Work out the finished part from the listing and answer in its coordinate system (mm). Face numbers are marked on the shaded views. A direction names the side the tool comes from. Coordinates: 2 decimals unless noted, no trailing zeros. Loops run counter-clockwise (first coordinate to the right, second up) from the corner with the lowest first, then second, coordinate; pieces in that order, holes last. Notation, with made-up numbers: (67, 88) -> (73, 88) arc R18 cw to (73, 112) -> close; hole circle Ø2 at (56.25, 11). An arc over 180 degrees is marked (long way). Answer as CSV lines item,"result".
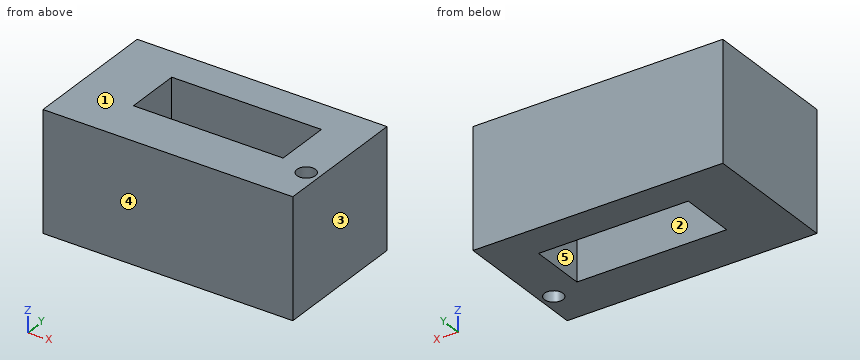
```python
from build123d import *

# Parameters (mm, degrees)
F0_W     = 53.355787
F0_H     = 29.385667
F0_R     = 1.970291
F0_W_2   = 31.967147
F0_H_2   = 11.958933
F1_DEPTH = 25.4


with BuildPart() as f1:
    # F0 (on Top) → F1 (new body)
    with BuildSketch(Plane.XY):
        with Locations((26.677893, 14.692833)):
            Rectangle(F0_W, F0_H)
        with Locations((50.581049, 8.259824)):
            Circle(F0_R, mode=Mode.SUBTRACT)
        with Locations((28.403014, 16.046856)):
            Rectangle(F0_W_2, F0_H_2, mode=Mode.SUBTRACT)
    extrude(amount=F1_DEPTH)


solid = f1.part
```
(1) A cutting plane is placed at B-B, the plane x = 41. Write down the section's boundary in (y, z), and give its area (3 significant figures).
Computed values:
outline,"(0, 0) -> (10.07, 0) -> (10.07, 25.4) -> (0, 25.4) -> close; (22.03, 0) -> (29.39, 0) -> (29.39, 25.4) -> (22.03, 25.4) -> close"
area,"443 mm2"
(2) Consider line 1 along Y through (x, z) = (19, 5.75); line 2 along X through (y, z) = (21.5, 20.5); line 3 along X through (y, z) = (8.75, 15.5). Determine where each line is inside the solid, lowest interval first.
Computed values:
line 1,"0 to 10.07, 22.03 to 29.39"
line 2,"0 to 12.42, 44.39 to 53.36"
line 3,"0 to 48.67, 52.49 to 53.36"
(3) A cutting plane is placed at C-C, the plane z = 15. Write down the section's boundary in (x, y).
Computed values:
outline,"(0, 0) -> (53.36, 0) -> (53.36, 29.39) -> (0, 29.39) -> close; hole (12.42, 10.07) -> (44.39, 10.07) -> (44.39, 22.03) -> (12.42, 22.03) -> close; hole circle Ø3.94 at (50.58, 8.26)"
(4) For a pull along X with two mould halves and no side action, classify the marked faces 3, 4 and 5 as pulls with the +X half, pulls with the -X half, needs draft (parallel to the pull), parting line crosses it, or undercut.
Computed values:
face 3,"pulls with the +X half"
face 4,"needs draft"
face 5,"undercut"
(5) Which of the six approach directions +Z, -Z, +X, -X, +Y, -Y give full straight-line access (tool end or side, diameter ignored) to the marked faces 1 and 2?
Computed values:
face 1,"+Z, +X, -X, +Y, -Y"
face 2,"+Z, -Z"
(6) A cutting plane is placed at A-A, the plane y = 17.75. Write down the section's boundary in (x, z).
Computed values:
outline,"(0, 0) -> (12.42, 0) -> (12.42, 25.4) -> (0, 25.4) -> close; (44.39, 0) -> (53.36, 0) -> (53.36, 25.4) -> (44.39, 25.4) -> close"
